For this review, use the dimensioned drawing (mm, ordinates from the lowest corner) and the shaded views. A direction names the side the tool comes from. Round coordinates to 2 decimals unless told otherwise and drop trailing zeros. Order: outer loops, then holes, each group sorted by start corner. A loop starts at its lowest first (then second) coordinate and runs counter-clockwise, first axis right, second up. Notation, with made-up numbers: (89, 14) -> (127, 14) arc R4 cw to (127, 19) -> close; hole circle Ø5 at (9, 5). An arc over 180 degrees is marked (long way). Use a Markdown table: item, result. Add a question column.
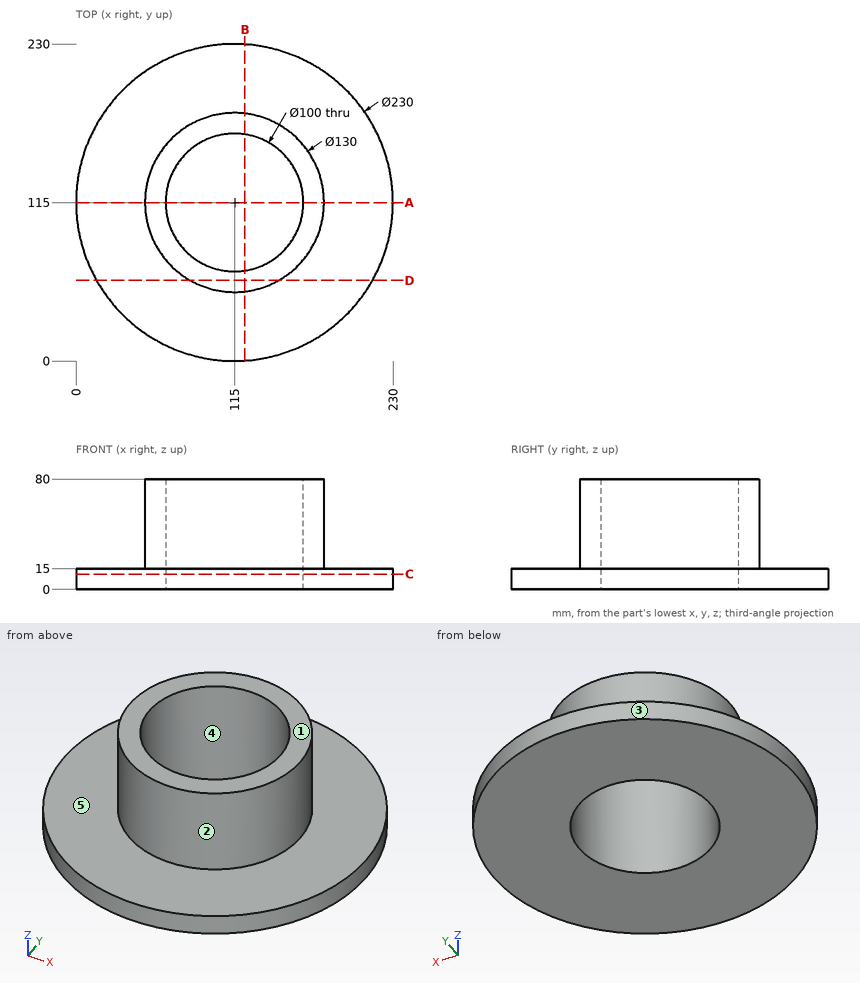
Q1. Add section D-D (y = 58.5). Write out the cut boundary in (x, z), then the cut area to 3 significant figures.
Q2. Add section A-A (y = 115). Write out the cut boundary in (x, z).
Q3. Wall thickness on line 1 (Y direction, x = 115, z = 17); line 2 (Z direction, x = 70.5, y = 51.5); line 3 (Y direction, x = 74, z = 51): over which ranges is each line inside the solid? List them lowest first. Write a range as [from, to].
Q4. Mouldability with a two-part tool opening along X and no side actions: class the marked faces 3, 4 and 5 as pulls with the +X half, pulls with the -X half, needs draft (parallel to the pull), parting line crosses it, or undercut.
Q5. Machinability: for the marked faces 1 and 2, which of the approach directions +Z, -Z, +X, -X, +Y, -Y give a long, thin tool a straight path to every point of the face, cutting with its end or side? Answer none if there is none.
Q6. Insertion check: pin 1 (1 mm diameter, centred on x = 83, z = 40, fed in from +Y); pin 2 (12 mm diameter, centred on x = 70.5, z = 55.5, fed in from -Y); pin 3 (2 mm diameter, centred on x = 106, y = 40, fed in from +Z). Each pin has a flat end and moves straight along its axis. Give the tip position at first contact, or say it passes through.
Q7. Add section C-C (z = 11). Write out the cut boundary in (x, y).
Q8. Add section B-B (x = 122.5). Write out the cut boundary in (y, z), then the cut area to 3 significant figures.
Report:
| question | item | result |
|---|---|---|
| 1 | outline | (14.84, 0) -> (215.16, 0) -> (215.16, 15) -> (147.14, 15) -> (147.14, 80) -> (82.86, 80) -> (82.86, 15) -> (14.84, 15) -> close |
| 1 | area | 7,180 mm² |
| 2 | outline | (0, 0) -> (65, 0) -> (65, 80) -> (50, 80) -> (50, 15) -> (0, 15) -> close; (165, 0) -> (230, 0) -> (230, 15) -> (180, 15) -> (180, 80) -> (165, 80) -> close |
| 3 | line 1 | y = [50, 65], [165, 180] |
| 3 | line 2 | z = [0, 15] |
| 3 | line 3 | y = [64.56, 86.38], [143.62, 165.44] |
| 4 | face 3 | parting line crosses it |
| 4 | face 4 | undercut |
| 4 | face 5 | needs draft |
| 5 | face 1 | +Z, +X, -X, +Y, -Y |
| 5 | face 2 | +Z |
| 6 | pin 1 | stops at y = 171.86 |
| 6 | pin 2 | stops at y = 62.63 |
| 6 | pin 3 | stops at z = 15 |
| 7 | outline | circle Ø230 at (115, 115); hole circle Ø100 at (115, 115) |
| 8 | outline | (0.24, 0) -> (65.57, 0) -> (65.57, 80) -> (50.43, 80) -> (50.43, 15) -> (0.24, 15) -> close; (164.43, 0) -> (229.76, 0) -> (229.76, 15) -> (179.57, 15) -> (179.57, 80) -> (164.43, 80) -> close |
| 8 | area | 3,930 mm² |
